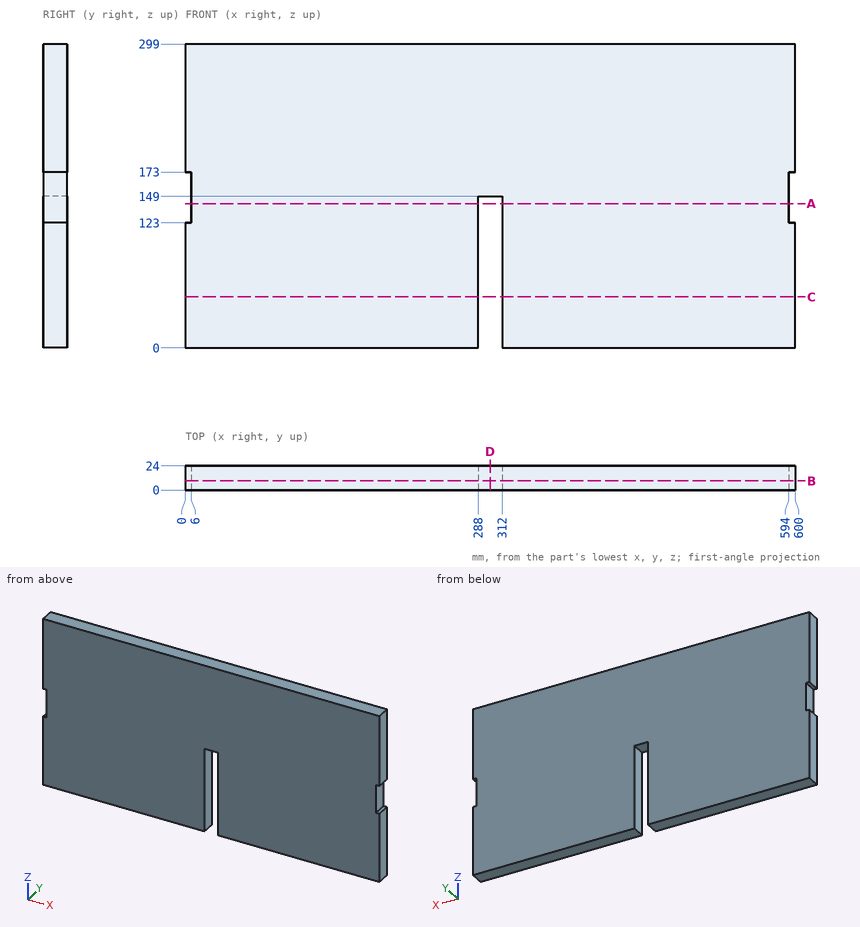
The drawing under review shows one solid part. Ordinate dimensions are in mm from its lowest x, y, z. Round coordinates to 2 decimals unless told otherwise and drop trailing zeros. Write each loop counter-clockwise with the first axis right and the second up, starting at its lowest first coordinate (ties: lowest second). Pieces come first, ordered by that corner, then holes. Notation, with made-up numbers: (59, -2) - (72, -2) arc R27 ccw to (72, 16) - close; hole circle Ø1 at (-25.5, 83). An arc over 180 degrees is marked (long way). Use a Markdown table: item, result. Add a question column.
1. Clearance check with flat-ended pins moving along their axes: pin 1 (2 mm diameter, centred on y = 15, z = 134, fed in from +X); pin 2 (12 mm diameter, centred on x = 295.5, y = 6.5, fed in from -Z). State where each tip first meets the part, or that it passes through.
2. Wall thickness on probe 1 along X at (y, z) = (3.25, 53); probe 2 along X at (y, z) = (10.75, 131): over which ranges is each line inside the solid? List them lowest first.
3. We need section D-D (x = 300). State the section outline as (y, z) points, then the cut area to 3 significant figures.
4. We need section C-C (z = 50). State the section outline as (x, y) points, then the cut area to 3 significant figures.
5. We need section B-B (y = 9.25). State the section outline as (x, z) points, then the cut area to 3 significant figures.
6. We need section A-A (z = 142). State the section outline as (x, y) points.
Output:
| question | item | result |
|---|---|---|
| 1 | pin 1 | stops at x = 594 |
| 1 | pin 2 | stops at z = 149 |
| 2 | probe 1 | x = 0 to 288, 312 to 600 |
| 2 | probe 2 | x = 6 to 288, 312 to 594 |
| 3 | outline | (0, 149) - (24, 149) - (24, 299) - (0, 299) - close |
| 3 | area | 3,600 mm2 |
| 4 | outline | (0, 0) - (288, 0) - (288, 24) - (0, 24) - close; (312, 0) - (600, 0) - (600, 24) - (312, 24) - close |
| 4 | area | 13,800 mm2 |
| 5 | outline | (0, 0) - (288, 0) - (288, 149) - (312, 149) - (312, 0) - (600, 0) - (600, 123) - (594, 123) - (594, 173) - (600, 173) - (600, 299) - (0, 299) - (0, 173) - (6, 173) - (6, 123) - (0, 123) - close |
| 5 | area | 175,000 mm2 |
| 6 | outline | (6, 0) - (288, 0) - (288, 24) - (6, 24) - close; (312, 0) - (594, 0) - (594, 24) - (312, 24) - close |
